The model under review builds one solid part; all positions refer to its coordinate system, in mm. Face numbers are marked on the shaded views. A direction names the side the tool comes from. Round coordinates to 2 decimals unless told otherwise and drop trailing zeros. Loops run counter-clockwise (first coordinate to the right, second up) from the corner with the lowest first, then second, coordinate; pieces in that order, holes last. Notation, with made-up numbers: M -39,23.25 L -19,23.25 A15 cw -19,48.25 Z; hole C 42,-31 d9. An arc over 180 degrees is marked long. Answer as a JSON object with one key per item and string values. Group by question number.
Item 1: To check wall thickness, follow line 1 (X direction, y = 28, z = 24.5); line 2 (Z direction, x = -23, y = 26). State the ranges of each line that lie inside material, in increasing order.
Item 2: Insertion check: P1, Ø8, axis at y = 26.5, z = 41.5, coming from the -X side; P2, Ø1.1, axis at x = -1, y = -36.5, coming from the -Z side; P3, Ø3, axis at x = -37, z = 39, coming from the +Y side; P4, Ø1.1, axis at x = 0, z = 74.5, coming from the -Y side. Each pin has a flat end and moves straight along its axis. Give the tip position at first contact, or say it passes through.
Item 3: The part is to be moulded in two halves that separate along X. For the marked faces 3, 4, 5 and 6, say which applies: +X half, -X half, draft (parallel to the pull), parting line (faces both ways), or undercut.
Item 4: Tool access review of the marked faces 1 and 2: name each direction out of +Z, -Z, +X, -X, +Y, -Y from which nothing blocks a thin tool from reaching the whole face with its end or side.
Item 5: Consider section D-D (z = 6.5). Give the boundary of the cut face in (x, y), and give its area (3 significant figures).
Item 6: Consider section B-B (x = 12.5). Give the boundary of the cut face in (y, z), and give its area (3 significant figures).
Item 7: Consider section A-A (z = 38). Give the boundary of the cut face in (x, y), and give its area (3 significant figures).
```python
from build123d import *

# Parameters (mm, degrees)
F0_W         = 76.2
F0_H         = 76.2
F1_DEPTH     = 76.2
F3_DEPTH     = 76.2
F5_DEPTH     = 76.2
F7_DEPTH     = 76.2
F8_T1_DEPTH  = 66.04
F8_T3_DEPTH  = 66.04
F8_T5_DEPTH  = 66.04
F8_S9_W      = 5.08
F8_S9_H      = 5.08
F8_T10_DEPTH = 5.08
F8_S15_W     = 5.08
F8_S15_H     = 5.08
F8_T16_DEPTH = 5.08
F8_S21_W     = 5.08
F8_S21_H     = 5.08
F8_T22_DEPTH = 5.08
F8_S27_W     = 5.08
F8_S27_H     = 5.08
F8_T28_DEPTH = 5.08
F8_S33_W     = 5.08
F8_S33_H     = 5.08
F8_T34_DEPTH = 5.08
F8_S39_W     = 5.08
F8_S39_H     = 5.08
F8_T40_DEPTH = 5.08
F8_S45_W     = 5.08
F8_S45_H     = 5.08
F8_T46_DEPTH = 5.08
F8_S51_W     = 5.08
F8_S51_H     = 5.08
F8_T52_DEPTH = 5.08
F9_R         = 5.08


# Not quite as in the source:
# - a fillet or chamfer that OpenCascade refuses, or shapes differently, is made with other operations: its cross-section is extruded or revolved along the edge and cut away or added


with BuildPart() as f1:
    # F0 (on Top) → F1 (new body)
    with BuildSketch(Plane.XY):
        Rectangle(F0_W, F0_H)
    extrude(amount=F1_DEPTH)

    # F2 (on face) → F3 (cut)
    with BuildSketch(Plane.XZ.offset(38.1)):
        Polygon((-3.81, 41.91), (-34.29, 41.91), (-34.29, 34.29), (-3.81, 34.29), (-3.81, 3.81), (3.81, 3.81), (3.81, 34.29), (34.29, 34.29), (34.29, 41.91), (3.81, 41.91), (3.81, 72.39), (-3.81, 72.39), align=None)
    extrude(amount=-F3_DEPTH, mode=Mode.SUBTRACT)

    # F4 (on face) → F5 (cut)
    with BuildSketch(Plane.XY.offset(76.2)):
        Polygon((3.81, 34.29), (-3.81, 34.29), (-3.81, 3.81), (-34.29, 3.81), (-34.29, -3.81), (-3.81, -3.81), (-3.81, -34.29), (3.81, -34.29), (3.81, -3.81), (34.29, -3.81), (34.29, 3.81), (3.81, 3.81), align=None)
    extrude(amount=-F5_DEPTH, mode=Mode.SUBTRACT)

    # F6 (on face) → F7 (cut)
    with BuildSketch(Plane.YZ.offset(38.1)):
        Polygon((-3.81, 41.91), (-34.29, 41.91), (-34.29, 34.29), (-3.81, 34.29), (-3.81, 3.81), (3.81, 3.81), (3.81, 34.29), (34.29, 34.29), (34.29, 41.91), (3.81, 41.91), (3.81, 72.39), (-3.81, 72.39), align=None)
    extrude(amount=-F7_DEPTH, mode=Mode.SUBTRACT)

    # F8: fillet of radius 5.08 on 12 edges, made by hand

    # F8_s2 → F8_t1 (cut)
    with BuildSketch(Plane.XY.offset(5.08)):
        with BuildLine():
            ThreePointArc((33.02, -38.1), (36.6121024484, -36.6121024484), (38.1, -33.02))
            Line((38.1, -33.02), (38.1, -38.1))
            Line((38.1, -38.1), (33.02, -38.1))
        make_face()
        with BuildLine():
            ThreePointArc((-33.02, -38.1), (-36.6121024484, -36.6121024484), (-38.1, -33.02))
            Line((-38.1, -33.02), (-38.1, -38.1))
            Line((-38.1, -38.1), (-33.02, -38.1))
        make_face()
        with BuildLine():
            ThreePointArc((33.02, 38.1), (36.6121024484, 36.6121024484), (38.1, 33.02))
            Line((38.1, 33.02), (38.1, 38.1))
            Line((38.1, 38.1), (33.02, 38.1))
        make_face()
        with BuildLine():
            ThreePointArc((-33.02, 38.1), (-36.6121024484, 36.6121024484), (-38.1, 33.02))
            Line((-38.1, 33.02), (-38.1, 38.1))
            Line((-38.1, 38.1), (-33.02, 38.1))
        make_face()
    extrude(amount=F8_T1_DEPTH, mode=Mode.SUBTRACT)

    # F8_s4 → F8_t3 (cut)
    with BuildSketch(Plane.YZ.offset(-33.02)):
        with BuildLine():
            ThreePointArc((-38.1, 71.12), (-36.6121024484, 74.7121024484), (-33.02, 76.2))
            Line((-33.02, 76.2), (-38.1, 76.2))
            Line((-38.1, 76.2), (-38.1, 71.12))
        make_face()
        with BuildLine():
            ThreePointArc((-38.1, 5.08), (-36.6121024484, 1.4878975516), (-33.02, 0))
            Line((-33.02, 0), (-38.1, 0))
            Line((-38.1, 0), (-38.1, 5.08))
        make_face()
        with BuildLine():
            ThreePointArc((38.1, 71.12), (36.6121024484, 74.7121024484), (33.02, 76.2))
            Line((33.02, 76.2), (38.1, 76.2))
            Line((38.1, 76.2), (38.1, 71.12))
        make_face()
        with BuildLine():
            ThreePointArc((38.1, 5.08), (36.6121024484, 1.4878975516), (33.02, 0))
            Line((33.02, 0), (38.1, 0))
            Line((38.1, 0), (38.1, 5.08))
        make_face()
    extrude(amount=F8_T3_DEPTH, mode=Mode.SUBTRACT)

    # F8_s6 → F8_t5 (cut)
    with BuildSketch(Plane.XZ.offset(-33.02)):
        with BuildLine():
            ThreePointArc((33.02, 76.2), (36.6121024484, 74.7121024484), (38.1, 71.12))
            Line((38.1, 71.12), (38.1, 76.2))
            Line((38.1, 76.2), (33.02, 76.2))
        make_face()
        with BuildLine():
            ThreePointArc((33.02, 0), (36.6121024484, 1.4878975516), (38.1, 5.08))
            Line((38.1, 5.08), (38.1, 0))
            Line((38.1, 0), (33.02, 0))
        make_face()
        with BuildLine():
            ThreePointArc((-38.1, 71.12), (-36.6121024484, 74.7121024484), (-33.02, 76.2))
            Line((-33.02, 76.2), (-38.1, 76.2))
            Line((-38.1, 76.2), (-38.1, 71.12))
        make_face()
        with BuildLine():
            ThreePointArc((-38.1, 5.08), (-36.6121024484, 1.4878975516), (-33.02, 0))
            Line((-33.02, 0), (-38.1, 0))
            Line((-38.1, 0), (-38.1, 5.08))
        make_face()
    extrude(amount=F8_T5_DEPTH, mode=Mode.SUBTRACT)


with BuildPart() as f8_tool8:
    # F8_s9 → F8_t10 (new body)
    with BuildSketch(Plane.XZ.offset(33.02)):
        with Locations((35.56, 2.54)):
            Rectangle(F8_S9_W, F8_S9_H)
    extrude(amount=F8_T10_DEPTH)

    # F8_s11 → F8_t12 (revolve, cut)
    with BuildSketch(Plane(origin=(33.02, -33.02, 5.08), x_dir=(-0.7071067812, 0, 0.7071067812), z_dir=(0.7071067812, 0, 0.7071067812))):
        with BuildLine():
            ThreePointArc((0, -5.08), (5.08, 0), (0, 5.08))
            Line((0, 5.08), (0, -5.08))
        make_face()
    revolve(axis=Axis((33.02, -33.02, 5.08), (0, -1, 0)), mode=Mode.SUBTRACT)


with BuildPart() as f1_1:
    add(f1.part)

    # F8_t7: cut F8_tool8
    add(f8_tool8.part, mode=Mode.SUBTRACT)


with BuildPart() as f8_tool14:
    # F8_s15 → F8_t16 (new body)
    with BuildSketch(Plane.XZ.offset(33.02)):
        with Locations((35.56, 73.66)):
            Rectangle(F8_S15_W, F8_S15_H)
    extrude(amount=F8_T16_DEPTH)

    # F8_s17 → F8_t18 (revolve, cut)
    with BuildSketch(Plane(origin=(33.02, -33.02, 71.12), x_dir=(-0.7071067812, 0, -0.7071067812), z_dir=(-0.7071067812, 0, 0.7071067812))):
        with BuildLine():
            ThreePointArc((0, -5.08), (5.08, 0), (0, 5.08))
            Line((0, 5.08), (0, -5.08))
        make_face()
    revolve(axis=Axis((33.02, -33.02, 71.12), (0, -1, 0)), mode=Mode.SUBTRACT)


with BuildPart() as f1_2:
    add(f1_1.part)

    # F8_t13: cut F8_tool14
    add(f8_tool14.part, mode=Mode.SUBTRACT)


with BuildPart() as f8_tool20:
    # F8_s21 → F8_t22 (new body)
    with BuildSketch(Plane.XZ.offset(33.02)):
        with Locations((-35.56, 73.66)):
            Rectangle(F8_S21_W, F8_S21_H)
    extrude(amount=F8_T22_DEPTH)

    # F8_s23 → F8_t24 (revolve, cut)
    with BuildSketch(Plane(origin=(-33.02, -33.02, 71.12), x_dir=(0.7071067812, 0, -0.7071067812), z_dir=(-0.7071067812, 0, -0.7071067812))):
        with BuildLine():
            ThreePointArc((0, -5.08), (5.08, 0), (0, 5.08))
            Line((0, 5.08), (0, -5.08))
        make_face()
    revolve(axis=Axis((-33.02, -33.02, 71.12), (0, -1, 0)), mode=Mode.SUBTRACT)


with BuildPart() as f1_3:
    add(f1_2.part)

    # F8_t19: cut F8_tool20
    add(f8_tool20.part, mode=Mode.SUBTRACT)


with BuildPart() as f8_tool26:
    # F8_s27 → F8_t28 (new body)
    with BuildSketch(Plane.XZ.offset(-33.02)):
        with Locations((35.56, 73.66)):
            Rectangle(F8_S27_W, F8_S27_H)
    extrude(amount=-F8_T28_DEPTH)

    # F8_s29 → F8_t30 (revolve, cut)
    with BuildSketch(Plane(origin=(33.02, 33.02, 71.12), x_dir=(-0.7071067812, 0, -0.7071067812), z_dir=(0.7071067812, 0, -0.7071067812))):
        with BuildLine():
            ThreePointArc((0, -5.08), (5.08, 0), (0, 5.08))
            Line((0, 5.08), (0, -5.08))
        make_face()
    revolve(axis=Axis((33.02, 33.02, 71.12), (0, 1, 0)), mode=Mode.SUBTRACT)


with BuildPart() as f1_4:
    add(f1_3.part)

    # F8_t25: cut F8_tool26
    add(f8_tool26.part, mode=Mode.SUBTRACT)


with BuildPart() as f8_tool32:
    # F8_s33 → F8_t34 (new body)
    with BuildSketch(Plane.XZ.offset(33.02)):
        with Locations((-35.56, 2.54)):
            Rectangle(F8_S33_W, F8_S33_H)
    extrude(amount=F8_T34_DEPTH)

    # F8_s35 → F8_t36 (revolve, cut)
    with BuildSketch(Plane(origin=(-33.02, -33.02, 5.08), x_dir=(0.7071067812, 0, 0.7071067812), z_dir=(0.7071067812, 0, -0.7071067812))):
        with BuildLine():
            ThreePointArc((0, -5.08), (5.08, 0), (0, 5.08))
            Line((0, 5.08), (0, -5.08))
        make_face()
    revolve(axis=Axis((-33.02, -33.02, 5.08), (0, -1, 0)), mode=Mode.SUBTRACT)


with BuildPart() as f1_5:
    add(f1_4.part)

    # F8_t31: cut F8_tool32
    add(f8_tool32.part, mode=Mode.SUBTRACT)


with BuildPart() as f8_tool38:
    # F8_s39 → F8_t40 (new body)
    with BuildSketch(Plane.XZ.offset(-33.02)):
        with Locations((35.56, 2.54)):
            Rectangle(F8_S39_W, F8_S39_H)
    extrude(amount=-F8_T40_DEPTH)

    # F8_s41 → F8_t42 (revolve, cut)
    with BuildSketch(Plane(origin=(33.02, 33.02, 5.08), x_dir=(-0.7071067812, 0, 0.7071067812), z_dir=(-0.7071067812, 0, -0.7071067812))):
        with BuildLine():
            ThreePointArc((0, -5.08), (5.08, 0), (0, 5.08))
            Line((0, 5.08), (0, -5.08))
        make_face()
    revolve(axis=Axis((33.02, 33.02, 5.08), (0, 1, 0)), mode=Mode.SUBTRACT)


with BuildPart() as f1_6:
    add(f1_5.part)

    # F8_t37: cut F8_tool38
    add(f8_tool38.part, mode=Mode.SUBTRACT)


with BuildPart() as f8_tool44:
    # F8_s45 → F8_t46 (new body)
    with BuildSketch(Plane.XZ.offset(-33.02)):
        with Locations((-35.56, 73.66)):
            Rectangle(F8_S45_W, F8_S45_H)
    extrude(amount=-F8_T46_DEPTH)

    # F8_s47 → F8_t48 (revolve, cut)
    with BuildSketch(Plane(origin=(-33.02, 33.02, 71.12), x_dir=(0.7071067812, 0, -0.7071067812), z_dir=(0.7071067812, 0, 0.7071067812))):
        with BuildLine():
            ThreePointArc((0, -5.08), (5.08, 0), (0, 5.08))
            Line((0, 5.08), (0, -5.08))
        make_face()
    revolve(axis=Axis((-33.02, 33.02, 71.12), (0, 1, 0)), mode=Mode.SUBTRACT)


with BuildPart() as f1_7:
    add(f1_6.part)

    # F8_t43: cut F8_tool44
    add(f8_tool44.part, mode=Mode.SUBTRACT)


with BuildPart() as f8_tool50:
    # F8_s51 → F8_t52 (new body)
    with BuildSketch(Plane.XZ.offset(-33.02)):
        with Locations((-35.56, 2.54)):
            Rectangle(F8_S51_W, F8_S51_H)
    extrude(amount=-F8_T52_DEPTH)

    # F8_s53 → F8_t54 (revolve, cut)
    with BuildSketch(Plane(origin=(-33.02, 33.02, 5.08), x_dir=(0.7071067812, 0, 0.7071067812), z_dir=(-0.7071067812, 0, 0.7071067812))):
        with BuildLine():
            ThreePointArc((0, -5.08), (5.08, 0), (0, 5.08))
            Line((0, 5.08), (0, -5.08))
        make_face()
    revolve(axis=Axis((-33.02, 33.02, 5.08), (0, 1, 0)), mode=Mode.SUBTRACT)


with BuildPart() as f1_8:
    add(f1_7.part)

    # F8_t49: cut F8_tool50
    add(f8_tool50.part, mode=Mode.SUBTRACT)

    # F9
    f9_edges = [f1_8.edges().sort_by_distance(p)[0] for p in [
        (3.81, 20.955, 34.29),
        (3.81, 20.955, 41.91),
        (-3.81, 20.955, 34.29),
        (-3.81, 20.955, 41.91),
        (20.955, 3.81, 34.29),
        (20.955, -3.81, 34.29),
        (20.955, -3.81, 41.91),
        (20.955, 3.81, 41.91),
        (-3.81, -20.955, 34.29),
        (-3.81, -20.955, 41.91),
        (3.81, -20.955, 34.29),
        (3.81, -20.955, 41.91),
        (-20.955, 3.81, 41.91),
        (-20.955, 3.81, 34.29),
        (-20.955, -3.81, 34.29),
        (-20.955, -3.81, 41.91),
    ]]
    fillet(f9_edges, radius=F9_R)


solid = f1_8.part
```
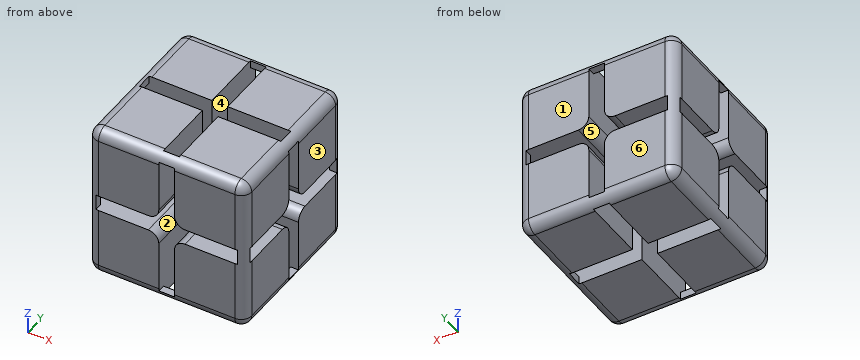
Geometry results:
{
 "1": {"line 1": "x = -38.1 to -3.81, 3.81 to 38.1", "line 2": "z = 0 to 34.29, 41.91 to 76.2"},
 "2": {"P1": "stops at x = -38.1", "P2": "stops at z = 0.93", "P3": "stops at y = 37.45", "P4": "stops at y = -37.24"},
 "3": {"face 3": "+X half", "face 4": "undercut", "face 5": "undercut", "face 6": "draft"},
 "4": {"face 1": "+Z, -Z, +X, -X, +Y", "face 2": "+Y, -Y"},
 "5": {"outline": "M -38.1,-33.02 A5.08 ccw -33.02,-38.1 L -3.81,-38.1 L -3.81,-3.81 L -38.1,-3.81 Z; M -38.1,3.81 L -3.81,3.81 L -3.81,38.1 L -33.02,38.1 A5.08 ccw -38.1,33.02 Z; M 3.81,-38.1 L 33.02,-38.1 A5.08 ccw 38.1,-33.02 L 38.1,-3.81 L 3.81,-3.81 Z; M 3.81,3.81 L 38.1,3.81 L 38.1,33.02 A5.08 ccw 33.02,38.1 L 3.81,38.1 Z", "area": "4,680 mm^2"},
 "6": {"outline": "M -38.1,5.08 A5.08 ccw -33.02,0 L -3.81,0 L -3.81,29.21 A5.08 ccw -8.89,34.29 L -38.1,34.29 Z; M -38.1,41.91 L -8.89,41.91 A5.08 ccw -3.81,46.99 L -3.81,76.2 L -33.02,76.2 A5.08 ccw -38.1,71.12 Z; M 3.81,0 L 33.02,0 A5.08 ccw 38.1,5.08 L 38.1,34.29 L 8.89,34.29 A5.08 ccw 3.81,29.21 Z; M 3.81,46.99 A5.08 ccw 8.89,41.91 L 38.1,41.91 L 38.1,71.12 A5.08 ccw 33.02,76.2 L 3.81,76.2 Z", "area": "4,660 mm^2"},
 "7": {"outline": "M -37.94,-34.29 A5.08 ccw -34.29,-37.94 L -34.29,-34.29 Z; M -37.94,34.29 L -34.29,34.29 L -34.29,37.94 A5.08 ccw Z; M 34.29,-37.94 A5.08 ccw 37.94,-34.29 L 34.29,-34.29 Z; M 34.29,34.29 L 37.94,34.29 A5.08 ccw 34.29,37.94 Z", "area": "36.5 mm^2"}
}
